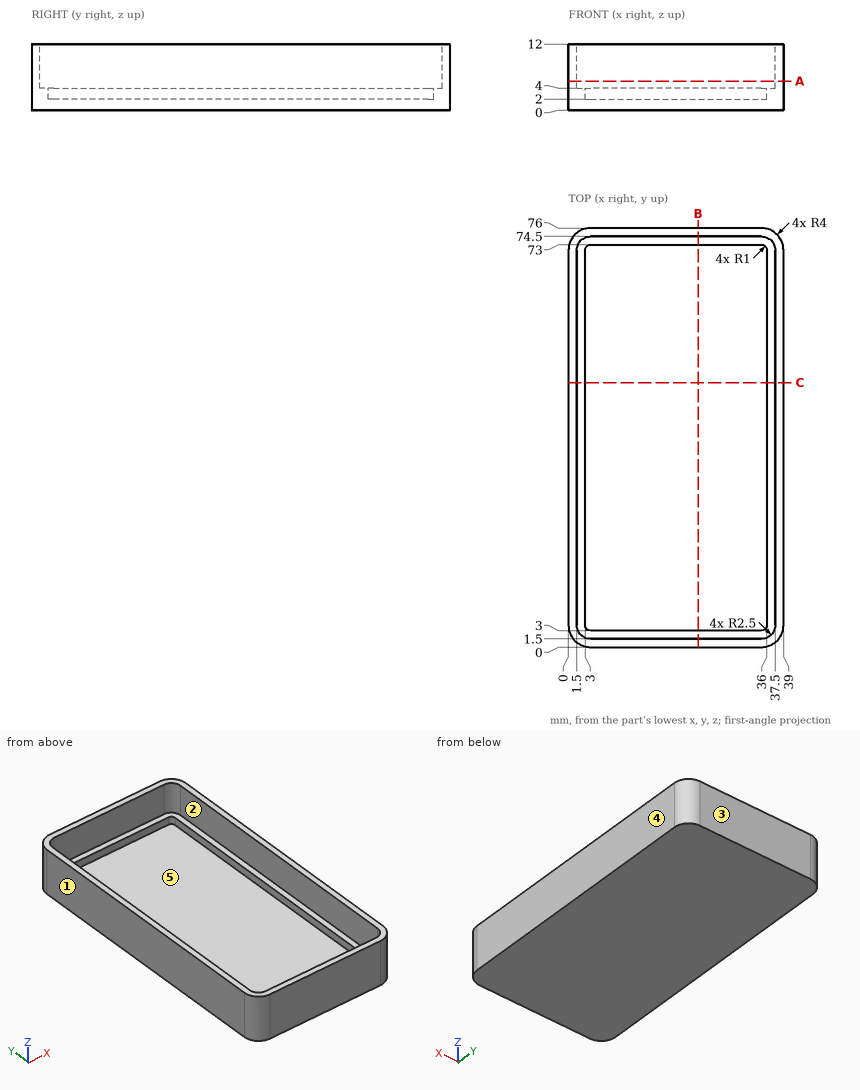
Design review of the part shown in the three views and the two pictorial views. Dimensions are in mm from the part's minimum x, y and z. A direction names the side the tool comes from. Round coordinates to 2 decimals unless told otherwise and drop trailing zeros. Write each loop counter-clockwise with the first axis right and the second up, starting at its lowest first coordinate (ties: lowest second). Pieces come first, ordered by that corner, then holes. Notation, with made-up numbers: M 44,-14 L 65,-14 A11 ccw 65,3 Z; hole C 17,80 d7. An arc over 180 degrees is marked long. One line per item, written item: value. Start each with the question number.
1. To check wall thickness, follow probe 1 along Y at (x, z) = (23, 5.25); probe 2 along X at (y, z) = (57, 8); probe 3 along X at (y, z) = (37.5, 3.5). State the ranges of each line that lie inside material, in increasing order. Write a range as from..to.
2. Take a section at A-A on z = 5.25. State the section outline as (x, y) points.
3. Take a section at C-C on y = 48. State the section outline as (x, z) points.
4. Draft analysis for pull direction X (two halves, no side actions). For the marked faces 1, 2 and 3, state which applies: pulls with the +X half, pulls with the -X half, needs draft (parallel to the pull), parting line crosses it, or undercut.
5. For the marked faces 4 and 5, list the 3-axis set-ups (+Z, -Z, +X, -X, +Y, -Y) from which the entire face can be reached by the end or side of a thin tool; tool diameter is ignored.
6. Take a section at B-B on x = 23.5. State the section outline as (y, z) points.
7. Clearance check with a flat-ended pin moving along its axis: P1, Ø16.5, axis at x = 22.5, y = 48, coming from the +Z side. State where the tip first meets the part, or that it passes through.
Computed:
1. probe 1: y = 0..1.5, 74.5..76
1. probe 2: x = 0..1.5, 37.5..39
1. probe 3: x = 0..3, 36..39
2. outline: M 0,4 A4 ccw 4,0 L 35,0 A4 ccw 39,4 L 39,72 A4 ccw 35,76 L 4,76 A4 ccw 0,72 Z; hole M 1.5,4 A2.5 ccw 4,1.5 L 35,1.5 A2.5 ccw 37.5,4 L 37.5,72 A2.5 ccw 35,74.5 L 4,74.5 A2.5 ccw 1.5,72 Z
3. outline: M 0,0 L 39,0 L 39,12 L 37.5,12 L 37.5,4 L 36,4 L 36,2 L 3,2 L 3,4 L 1.5,4 L 1.5,12 L 0,12 Z
4. face 1: pulls with the -X half
4. face 2: undercut
4. face 3: needs draft
5. face 4: +Z, -Z, +X, +Y, -Y
5. face 5: +Z
6. outline: M 0,0 L 76,0 L 76,12 L 74.5,12 L 74.5,4 L 73,4 L 73,2 L 3,2 L 3,4 L 1.5,4 L 1.5,12 L 0,12 Z
7. P1: stops at z = 2
